from build123d import *

# Parameters (mm, degrees)
SKETCH1_R           = 62.5
SKETCH1_R_2         = 57.5
BOSS_EXTRUDE1_DEPTH = 10
SKETCH2_R           = 62.5
BOSS_EXTRUDE2_DEPTH = 22
SKETCH3_R           = 1.5
CUT_EXTRUDE1_DEPTH  = 92.08512502
SKETCH4_W           = 100
SKETCH4_H           = 100
CUT_EXTRUDE2_DEPTH  = 16
SKETCH6_R           = 6
CUT_EXTRUDE3_DEPTH  = 3


with BuildPart() as part:
    # Sketch1 → Boss-Extrude1 (new body)
    with BuildSketch(Plane.XY):
        Circle(SKETCH1_R)
        Circle(SKETCH1_R_2, mode=Mode.SUBTRACT)
    extrude(amount=BOSS_EXTRUDE1_DEPTH)

    # Sketch2 → Boss-Extrude2 (add)
    with BuildSketch(Plane.XY.offset(10)):
        Circle(SKETCH2_R)
    extrude(amount=BOSS_EXTRUDE2_DEPTH)

    # Sketch3 → Cut-Extrude1 (cut, through all)
    with BuildSketch(Plane(origin=(0, 0, 10), x_dir=(-1, 0, 0), z_dir=(0, 0, -1))):
        Circle(SKETCH3_R)
    extrude(amount=-CUT_EXTRUDE1_DEPTH, mode=Mode.SUBTRACT)

    # Sketch4 → Cut-Extrude2 (cut)
    with BuildSketch(Plane.XY.offset(32)):
        with Locations((33, 0)):
            Rectangle(SKETCH4_W, SKETCH4_H)
    extrude(amount=-CUT_EXTRUDE2_DEPTH, mode=Mode.SUBTRACT)

    # Sketch6 → Cut-Extrude3 (cut)
    with BuildSketch(Plane.XY.offset(16)):
        Circle(SKETCH6_R)
    extrude(amount=-CUT_EXTRUDE3_DEPTH, mode=Mode.SUBTRACT)


solid = part.part
Model file for the job. Use its own axes, mm. A direction names the side the tool comes from. Give positions to 0.01 mm unless a question says otherwise; leave off trailing zeros. Order: outer loops, then holes, each group sorted by start corner. A loop starts at its lowest first (then second) coordinate and runs counter-clockwise, first axis right, second up. Notation, with made-up numbers: (51, 45) -> (71, 45) arc R12 ccw to (71, 55) -> close; hole circle Ø2 at (45.5, 68). An arc over 180 degrees is marked (long way). Use CSV: the item, a comma, the result in double quotes.
1. Drill centre lines: line 1 along Y through (x, z) = (0, 4.5); line 2 along Y through (x, z) = (0, 12); line 3 along X through (y, z) = (-12.5, 2.5). Where is each one in solid material? Low to high. Write a range as from..to.
Outcome:
line 1,"-62.5..-57.5, 57.5..62.5"
line 2,"-62.5..-1.5, 1.5..62.5"
line 3,"-61.24..-56.12, 56.12..61.24"
2. Band-saw the part on B-B, the plane x = 0. Give the cut face in (y, z), then the cut area to 4 significant figures.
Outcome:
outline,"(-62.5, 0) -> (-57.5, 0) -> (-57.5, 10) -> (-1.5, 10) -> (-1.5, 13) -> (-6, 13) -> (-6, 16) -> (-50, 16) -> (-50, 32) -> (-62.5, 32) -> close; (1.5, 10) -> (57.5, 10) -> (57.5, 0) -> (62.5, 0) -> (62.5, 32) -> (50, 32) -> (50, 16) -> (6, 16) -> (6, 13) -> (1.5, 13) -> close"
area,"1,205 mm²"
3. Band-saw the part on C-C, the plane z = 4. Give the cut face in (x, y).
Outcome:
outline,"circle Ø125 at (0, 0); hole circle Ø115 at (0, 0)"
4. 3-axis set-ups, long thin cutter, end or side, ignore diameter. For faces 5 (the flat face through (10, -50, 24)), 6 (the cylindrical face through (-6, 0, 15)), 7 (the flat face through (27, -51, 0)), 8 (the flat face through (-24, 1, 32)), 9 (the cylindrical face through (-12.465, -56.133, 4.93)): which of +Z, -Z, +X, -X, +Y, -Y reach the whole face in a straight line?
Outcome:
face 5,"+Z, +X"
face 6,"+Z"
face 7,"-Z, +X, -X, +Y, -Y"
face 8,"+Z, +X, -X, +Y, -Y"
face 9,"-Z"
5. Drop flat-ended pins along their axis: pin 1 (1.5 mm diameter, centred on x = 38, z = 20, fed in from +Y); pin 2 (3 mm diameter, centred on x = -14.5, y = 24.5, fed in from -Z); pin 3 (12 mm diameter, centred on y = -49, z = 3.5, fed in from -X). Give the stop position or say it passes through.
Outcome:
pin 1,"y = 50.19"
pin 2,"z = 10"
pin 3,"x = -45.36"
6. Mould opens along X. For faces 1 (the cylindrical face through (-62.44, 2.75, 15.78)), 2 (the flat face through (12, 1, 10)), 3 (the flat face through (22, 1, 16)), 4 (the cylindrical face through (1.5, 0.07, 11.48)) say: +X half, -X half, draft (parallel to the pull), parting line (faces both ways), or undercut.
Outcome:
face 1,"parting line"
face 2,"undercut"
face 3,"draft"
face 4,"undercut"
7. Band-saw the part on A-A, the plane y = 0. Give the cut face in (x, z).
Outcome:
outline,"(-62.5, 0) -> (-57.5, 0) -> (-57.5, 10) -> (-1.5, 10) -> (-1.5, 13) -> (-6, 13) -> (-6, 16) -> (-17, 16) -> (-17, 32) -> (-62.5, 32) -> close; (1.5, 10) -> (57.5, 10) -> (57.5, 0) -> (62.5, 0) -> (62.5, 16) -> (6, 16) -> (6, 13) -> (1.5, 13) -> close"
8. Band-saw the part on D-D, the plane y = 25. Give the cut face in (x, z).
Outcome:
outline,"(-57.28, 0) -> (-51.78, 0) -> (-51.78, 10) -> (51.78, 10) -> (51.78, 0) -> (57.28, 0) -> (57.28, 16) -> (-17, 16) -> (-17, 32) -> (-57.28, 32) -> close"
